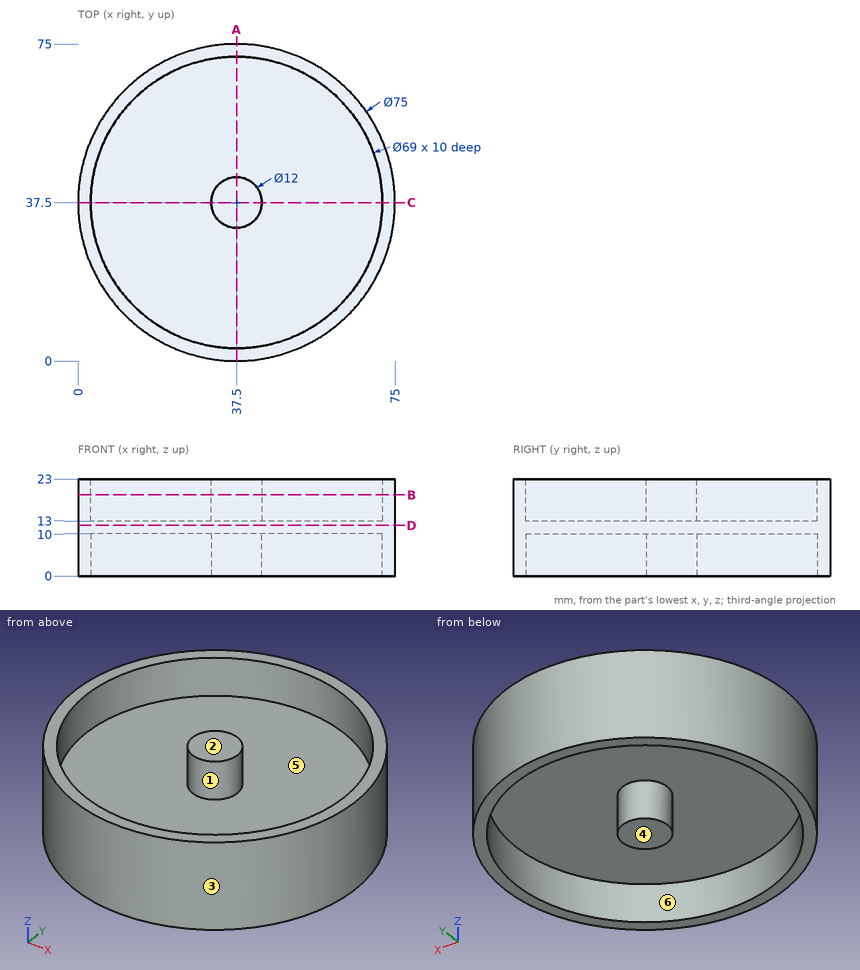
Here's the drawing with two shaded views (mm, measured from the low corner). I have some questions. A direction names the side the tool comes from. Give positions to 0.01 mm unless a question says otherwise; leave off trailing zeros. Loops run counter-clockwise (first coordinate to the right, second up) from the corner with the lowest first, then second, coordinate; pieces in that order, holes last. Notation, with made-up numbers: M 64,2.25 L 110,2.25 A24 ccw 110,17.25 Z; hole C -31,-40 d4. An arc over 180 degrees is marked long. Answer in a Markdown table with one row per item.
1. Thinking about a two-plate mould opening in Y: for the marked faces 1, 2 and 3, which applies, released by +Y, released by -Y, zero draft, split by the parting line, or undercut?
Taken from the geometry:
| item | result |
|---|---|
| face 1 | undercut |
| face 2 | zero draft |
| face 3 | split by the parting line |
2. Suppose I cut it at A-A on x = 37.5. Write out the boundary of the cut face in (y, z).
Taken from the geometry:
| item | result |
|---|---|
| outline | M 0,0 L 3,0 L 3,10 L 31.5,10 L 31.5,0 L 43.5,0 L 43.5,10 L 72,10 L 72,0 L 75,0 L 75,23 L 72,23 L 72,13 L 43.5,13 L 43.5,23 L 31.5,23 L 31.5,13 L 3,13 L 3,23 L 0,23 Z |
3. Suppose I cut it at D-D on z = 12. Write out the boundary of the cut face in (x, y), plus the area to 3 significant figures.
Taken from the geometry:
| item | result |
|---|---|
| outline | C 37.5,37.5 d75 |
| area | 4,420 mm² |
4. Which directions (+Z, -Z, +X, -X, +Y, -Y) give clear straight access to the entire face, cutting with the end or side of a thin tool? Please do the marked faces 4, 5 and 6.
Taken from the geometry:
| item | result |
|---|---|
| face 4 | -Z, +X, -X, +Y, -Y |
| face 5 | +Z |
| face 6 | -Z |
5. Suppose I cut it at B-B on z = 19.25. Write out the boundary of the cut face in (x, y), plus the area to 3 significant figures.
Taken from the geometry:
| item | result |
|---|---|
| outline | C 37.5,37.5 d75; C 37.5,37.5 d12; hole C 37.5,37.5 d69 |
| area | 792 mm² |
6. For pin 1 Ø1.5 at (y, z) = (52, 5) entering from -X; pin 2 Ø1.5 at (y, z) = (51, 3) entering from -X; pin 3 Ø3 at (x, z) = (41.5, 4) entering from -Y, each with a flat end and sliding along its axis, tell me the tip position at first contact or that it passes through.
Taken from the geometry:
| item | result |
|---|---|
| pin 1 | stops at x = 2.61 |
| pin 2 | stops at x = 2.23 |
| pin 3 | stops at y = 0.08 |
7. If I drill on line 1 along Y through (x, z) = (37.5, 2); line 2 along Y through (x, z) = (33, 2.25); line 3 along Z through (x, y) = (26, 16.5), over which ranges is the centre line in solid material (lowest first)?
Taken from the geometry:
| item | result |
|---|---|
| line 1 | y = 0 to 3, 31.5 to 43.5, 72 to 75 |
| line 2 | y = 0.27 to 3.29, 33.53 to 41.47, 71.71 to 74.73 |
| line 3 | z = 10 to 13 |
